Geometry check sheet. Reference: the model listing, model coordinates, mm. A direction names the side the tool comes from. Give positions to 0.01 mm unless a question says otherwise; leave off trailing zeros. Write each loop counter-clockwise with the first axis right and the second up, starting at its lowest first coordinate (ties: lowest second). Pieces come first, ordered by that corner, then holes. Notation, with made-up numbers: M 0,-1.5 L 7,-1.5 A15 ccw 7,2.5 Z; hole C 18,79 d7. An arc over 180 degrees is marked long. One line per item, written item: value. Start each with the question number.
1. Cross-section at D-D on z = -10. Record the cut outline in (x, y), then the cut area to 3 significant figures.
2. Gauge pin test, flat ends, axial feed: pin 1 (4 mm diameter, centred on x = 3.5, y = 16.5, fed in from -Z); pin 2 (6 mm diameter, centred on x = 1.5, z = 16.5, fed in from +Y); pin 3 (2 mm diameter, centred on x = 4, y = 18.5, fed in from +Z). Record the tip position at first contact, or that the pin passes through.
3. Cross-section at C-C on z = 0. Record the cut outline in (x, y), then the cut area to 3 significant figures.
4. Scan lines: line 1 (Z direction, x = 3.5, y = 9.5); line 2 (Z direction, x = 6, y = 7.3); line 3 (Y direction, x = 2.5, z = -7). Record each from-to range of solid material in increasing order.
5. Tool access check on faces 5 (the face through (6, 16, 10.8)), 6 (the face through (3, 8, 0)), 7 (the face through (11.5, 3.9, 22)). Record the directions out of +Z, -Z, +X, -X, +Y, -Y that give a thin tool (end or side, any length) a straight path to the whole face; none if there is none.
6. Cross-section at A-A on y = 13. Record the cut outline in (x, z).
7. Cross-section at B-B on x = 6. Record the cut outline in (y, z).
8. Release check for a two-part mould opening along Z. For faces 1 (the face through (6, 15, -10.8)), 2 (the face through (11.5, 3.9, -20)), 3 (the face through (6, 16, -7.8)), 4 (the face through (1, 0, 0)) record: pulls with the +Z half, pulls with the -Z half, needs draft (parallel to the pull), parting line crosses it, or undercut.
from build123d import *

# Parameters (mm, degrees)
BOSS_EXTRUDE1_DEPTH                              = 12
CBORE_FOR_M4_PAN_HEAD_MACHINE_SCREW1_D           = 4.8
CBORE_FOR_M4_PAN_HEAD_MACHINE_SCREW1_CBORE_D     = 9
CBORE_FOR_M4_PAN_HEAD_MACHINE_SCREW1_CBORE_DEPTH = 7
F_6_0MM_DOWEL_HOLE1_D                            = 6.2
SKETCH13_W                                       = 1
SKETCH13_H                                       = 2
CUT_EXTRUDE1_DEPTH                               = 12


with BuildPart() as part:
    # Sketch4 → Boss-Extrude1 (new body)
    with BuildSketch(Plane(origin=(0, 0, 0), x_dir=(0, 0, -1), z_dir=(1, 0, 0))):
        Polygon((-25, 0), (0, 0), (0, 8), (-7.8, 8), (-7.8, 23), (-10.8, 23), (-10.8, 8), (-25, 8), align=None)
        Polygon((0, 8), (0, 0), (25, 0), (25, 8), (10.8, 8), (10.8, 23), (7.8, 23), (7.8, 8), align=None)
    extrude(amount=BOSS_EXTRUDE1_DEPTH)

    # CBORE for M4 Pan Head Machine Screw1 (through all)
    with Locations(Plane(origin=(0, 0, 0), x_dir=(-1, 0, 0), z_dir=(0, -1, 0))):
        with Locations((-6, 0)):
            CounterBoreHole(CBORE_FOR_M4_PAN_HEAD_MACHINE_SCREW1_D / 2, CBORE_FOR_M4_PAN_HEAD_MACHINE_SCREW1_CBORE_D / 2, CBORE_FOR_M4_PAN_HEAD_MACHINE_SCREW1_CBORE_DEPTH)

    # Ø6.0mm Dowel Hole1 (through all)
    with Locations(Plane.XY.offset(25)):
        with Locations((6, 0)):
            Hole(F_6_0MM_DOWEL_HOLE1_D / 2)

    # Sketch13 → Cut-Extrude1 (cut)
    with BuildSketch(Plane.XZ):
        with Locations((0.5, -21)):
            Rectangle(SKETCH13_W, SKETCH13_H)
        with Locations((0.5, 21)):
            Rectangle(SKETCH13_W, SKETCH13_H)
        with Locations((11.5, 21)):
            Rectangle(SKETCH13_W, SKETCH13_H)
        with Locations((11.5, -21)):
            Rectangle(SKETCH13_W, SKETCH13_H)
    extrude(amount=-CUT_EXTRUDE1_DEPTH, mode=Mode.SUBTRACT)


solid = part.part
Report:
1. outline: M 0,0 L 2.9,0 A3.1 cw 9.1,0 L 12,0 L 12,23 L 0,23 Z
1. area: 261 mm^2
2. pin 1: stops at z = -10.8
2. pin 2: stops at y = 8
2. pin 3: stops at z = 10.8
3. outline: M 0,0 L 1.5,0 L 1.5,7 L 3.6,7 L 3.6,8 L 0,8 Z; M 8.4,7 L 10.5,7 L 10.5,0 L 12,0 L 12,8 L 8.4,8 Z
3. area: 28.2 mm^2
4. line 1: z = -10.8 to -7.8, 7.8 to 10.8
4. line 2: z = -25 to -2.4, 2.4 to 25
4. line 3: y = 0 to 8
5. face 5: +Z, +X, -X, +Y
5. face 6: +X, -X, +Y
5. face 7: +X, +Y, -Y
6. outline: M 0,-10.8 L 12,-10.8 L 12,-7.8 L 0,-7.8 Z; M 0,7.8 L 12,7.8 L 12,10.8 L 0,10.8 Z
7. outline: M 3.1,-25 L 8,-25 L 8,-10.8 L 23,-10.8 L 23,-7.8 L 8,-7.8 L 8,-2.4 L 7,-2.4 L 7,-4.5 L 3.1,-4.5 Z; M 3.1,4.5 L 7,4.5 L 7,2.4 L 8,2.4 L 8,7.8 L 23,7.8 L 23,10.8 L 8,10.8 L 8,25 L 3.1,25 Z
8. face 1: pulls with the -Z half
8. face 2: undercut
8. face 3: undercut
8. face 4: needs draft
